from build123d import *

# Parameters (mm, degrees)
BOSS_EXTRUDE1_DEPTH = 25.0444
CUT_EXTRUDE1_DEPTH  = 60.520050184
LPATTERN1_COUNT     = 11
LPATTERN1_PITCH     = 3.175
CUT_EXTRUDE2_DEPTH  = 60.520050184
FILLET1_R           = 1.905


with BuildPart() as part:
    # Sketch1 → Boss-Extrude1 (new body)
    with BuildSketch(Plane.XY):
        Polygon((0, 0), (52.07, 0), (52.658318987, 1.811473978), (46.811766462, 11.938), (-11.476681013, 11.938), (-11.476681013, 6.35), align=None)
    extrude(amount=BOSS_EXTRUDE1_DEPTH)

    # Sketch2 → Cut-Extrude1 (cut, through all)
    with BuildSketch(Plane.XY.offset(25.0444)):
        Polygon((51.070818987, 4.561104635), (50.181267753, 1.249497834), (52.658318987, 1.811473978), align=None)
    cut_extrude1 = extrude(amount=-CUT_EXTRUDE1_DEPTH, mode=Mode.SUBTRACT)

    # LPattern1: Cut-Extrude1 ×11
    with Locations(*[Vector(-0.49999999999999795, 0.8660254037844398, 0) * (i * LPATTERN1_PITCH) for i in range(1, LPATTERN1_COUNT)]):
        add(cut_extrude1, mode=Mode.SUBTRACT)

    # Sketch3 → Cut-Extrude2 (cut, through all)
    with BuildSketch(Plane(origin=(0, 11.938, 0), x_dir=(1, 0, 0), z_dir=(0, 1, 0))):
        with BuildLine():
            Line((10.494318987, -6.2992), (26.623318987, -6.2992))
            ThreePointArc((26.623318987, -6.2992), (32.846318987, -12.5222), (26.623318987, -18.7452))
            Line((26.623318987, -18.7452), (10.494318987, -18.7452))
            ThreePointArc((10.494318987, -18.7452), (4.271318987, -12.5222), (10.494318987, -6.2992))
        make_face()
        Polygon((-11.476681013, -6.1722), (-0.046681013, 0), (-11.476681013, 0), align=None)
        Polygon((-11.476681013, -25.0444), (-0.046681013, -25.0444), (-11.476681013, -18.8722), align=None)
    extrude(amount=-CUT_EXTRUDE2_DEPTH, mode=Mode.SUBTRACT)

    # Fillet1
    fillet1_edges = [part.edges().sort_by_distance(p)[0] for p in [
        (23.013702779, 11.938, 25.0444),
        (23.013702779, 11.938, 0),
        (26.035, 0, 0),
        (26.035, 0, 25.0444),
    ]]
    fillet(fillet1_edges, radius=FILLET1_R)


solid = part.part
Read the model definition and answer for the solid it produces. Units are mm, in the model's axes. A direction names the side the tool comes from. Give positions to 0.01 mm unless a question says otherwise; leave off trailing zeros. Loops run counter-clockwise (first coordinate to the right, second up) from the corner with the lowest first, then second, coordinate; pieces in that order, holes last. Notation, with made-up numbers: M -2,53 L 41,53 A17 ccw 41,74 Z; hole C 18,57.5 d7. An arc over 180 degrees is marked long. Write each question's results on one line, items separated by ' | '.
1. Given pin 1 (3 mm diameter, centred on y = 4, z = 6, fed in from -X); pin 2 (1 mm diameter, centred on y = 4, z = 20, fed in from -X), each flat-ended and moving along its own axis, determine where each tip first touches the part or whether it passes through.
Values:
pin 1: stops at x = -9.94 | pin 2: stops at x = -8.13
2. Section D-D on z = 4 is taken. Give the vertices of the cut face in (x, y).
Values:
outline: M -7.45,4.12 L 0,0 L 52.07,0 L 52.66,1.81 L 50.18,1.25 L 51.07,4.56 L 48.59,4 L 49.48,7.31 L 47.01,6.75 L 47.9,10.06 L 45.42,9.5 L 46.07,11.94 L -7.45,11.94 Z
3. Section C-C on y = 10.75 is taken. Give the vertices of the cut face in (x, z).
Values:
outline: M -11.48,6.17 L -0.31,0.14 L 45.75,0.14 L 45.75,24.9 L -0.31,24.9 L -11.48,18.87 Z; hole M 10.49,6.3 L 26.62,6.3 A6.22 ccw 26.62,18.75 L 10.49,18.75 A6.22 ccw Z
4. Straight lines are drawn through the part: line 1 (Z direction, x = 17, y = 2.75); line 2 (Z direction, x = 9.5, y = 6.5); line 3 (X direction, y = 7.5, z = 8.25). For each, find the intervals that lie inside material, in ascending order. Write a range as [from, to].
Values:
line 1: z = [0, 6.3], [18.75, 25.04] | line 2: z = [0, 6.38], [18.67, 25.04] | line 3: x = [-11.48, 5.97], [31.15, 47.21]
5. Section B-B on z = 15 is taken. Give the vertices of the cut face in (x, y).
Values:
outline: M -11.48,6.35 L 0,0 L 4.79,0 L 4.79,11.94 L -11.48,11.94 Z; M 32.33,0 L 52.07,0 L 52.66,1.81 L 50.18,1.25 L 51.07,4.56 L 48.59,4 L 49.48,7.31 L 47.01,6.75 L 47.9,10.06 L 45.42,9.5 L 46.07,11.94 L 32.33,11.94 Z
6. Section A-A on x = 24 is taken. Give the vertices of the cut face in (y, z) (3 decimals), plus the area to 3 significant figures.
Values:
outline: M 0,1.905 A1.905 ccw 1.905,0 L 10.033,0 A1.905 ccw 11.938,1.905 L 11.938,6.299 L 0,6.299 Z; M 0,18.745 L 11.938,18.745 L 11.938,23.139 A1.905 ccw 10.033,25.044 L 1.905,25.044 A1.905 ccw 0,23.139 Z | area: 147 mm^2
7. A tool of negligible diameter and unlimited length cuts with its end or side. For faces 1 (the face through (18, 11.938, 19)), 2 (the face through (18, 6, 6.299)), 3 (the face through (49.815, 4.276, 12.698)), from which of +Z, -Z, +X, -X, +Y, -Y can it reach the whole face along a straight path? Write none if from no direction.
Values:
face 1: +Z, -Z, +X, -X, +Y | face 2: +Y, -Y | face 3: +Z, -Z
8. The mould has two halves that part along Z. Classify faces 4 (the face through (48.227, 7.026, 12.698)), 5 (the face through (19, 6, 18.745)), 6 (the face through (20.902, 11.365, 0.543)): pulls with the +Z half, pulls with the -Z half, needs draft (parallel to the pull), parting line crosses it, or undercut.
Values:
face 4: needs draft | face 5: undercut | face 6: pulls with the -Z half
